Here's how the part is built. I have some questions about the finished solid (model axes, mm). A direction names the side the tool comes from. Round coordinates to 2 decimals unless told otherwise and drop trailing zeros. Order: outer loops, then holes, each group sorted by start corner. A loop starts at its lowest first (then second) coordinate and runs counter-clockwise, first axis right, second up. Notation, with made-up numbers: M -37,63 L 5,63 A14 cw 5,88 Z; hole C 69.25,45 d6. An arc over 180 degrees is marked long. Answer as CSV lines item,"result". Start each with the question number.
```python
from build123d import *

# Parameters (mm, degrees)
SKETCH_1_R          = 5
SKETCH_1_R_2        = 3
EXTRUDE_1_DEPTH     = 12
SKETCH_2_R          = 5.5
CUT_EXTRUDE_1_DEPTH = 6


with BuildPart() as part:
    # 草图1 → 凸台-拉伸1 (new body)
    with BuildSketch(Plane.XY):
        with BuildLine():
            Line((-35, 0), (-35, 35))
            Line((-35, 35), (35, 35))
            Line((35, 35), (35, 0))
            ThreePointArc((35, 0), (0, -35), (-35, 0))
        make_face()
        Circle(SKETCH_1_R, mode=Mode.SUBTRACT)
        with Locations((-27, 29)):
            Circle(SKETCH_1_R_2, mode=Mode.SUBTRACT)
        with Locations((-9, 29)):
            Circle(SKETCH_1_R_2, mode=Mode.SUBTRACT)
        with Locations((9, 29)):
            Circle(SKETCH_1_R_2, mode=Mode.SUBTRACT)
        with Locations((27, 29)):
            Circle(SKETCH_1_R_2, mode=Mode.SUBTRACT)
        with BuildLine():
            ThreePointArc((30, 0), (27, 3), (24, 0))
            ThreePointArc((24, 0), (0, -24), (-24, 0))
            ThreePointArc((-24, 0), (-27, 3), (-30, 0))
            ThreePointArc((-30, 0), (0, -30), (30, 0))
        make_face(mode=Mode.SUBTRACT)
        with BuildLine():
            ThreePointArc((17, 0), (14, 3), (11, 0))
            ThreePointArc((11, 0), (0, -11), (-11, 0))
            ThreePointArc((-11, 0), (-14, 3), (-17, 0))
            ThreePointArc((-17, 0), (0, -17), (17, 0))
        make_face(mode=Mode.SUBTRACT)
    extrude(amount=EXTRUDE_1_DEPTH)

    # 草图2 → 切除-拉伸1 (cut)
    with BuildSketch(Plane.XY.offset(12)):
        with Locations((-27, 29)):
            Circle(SKETCH_2_R)
        with Locations((-9, 29)):
            Circle(SKETCH_2_R)
        with Locations((9, 29)):
            Circle(SKETCH_2_R)
        with Locations((27, 29)):
            Circle(SKETCH_2_R)
        with BuildLine():
            ThreePointArc((32.5, 0), (27, 5.5), (21.5, 0))
            ThreePointArc((21.5, 0), (0, -21.5), (-21.5, 0))
            ThreePointArc((-21.5, 0), (-27, 5.5), (-32.5, 0))
            ThreePointArc((-32.5, 0), (0, -32.5), (32.5, 0))
        make_face()
        with BuildLine():
            ThreePointArc((19.5, 0), (14, 5.5), (8.5, 0))
            ThreePointArc((8.5, 0), (0, -8.5), (-8.5, 0))
            ThreePointArc((-8.5, 0), (-14, 5.5), (-19.5, 0))
            ThreePointArc((-19.5, 0), (0, -19.5), (19.5, 0))
        make_face()
    extrude(amount=-CUT_EXTRUDE_1_DEPTH, mode=Mode.SUBTRACT)


solid = part.part
```
Item 1: If I drill on line 1 along X through (y, z) = (29, 4.5); line 2 along Y through (x, z) = (0, 6.25); line 3 along Y through (x, z) = (0, 3.25), over which ranges is the centre line in solid material (lowest first)?
Item 2: If we section it at C-C on y = -25: Please give me the cut outline in (x, z).
Item 3: If we section it at D-D on y = 29: Count the separate pieces of the cut face and the enclosed holes in it, and give its area (3 significant figures).
Item 4: If we section it at A-A on x = 0: Please give me the cut outline in (y, z).
Item 5: For P1, Ø4, axis at x = -8.5, z = 3, coming from the -Y side; P2, Ø3.5, axis at x = 29, y = 30, coming from the +Z side; P3, Ø6, axis at x = -23, z = 6, coming from the -Y side, each with a flat end and sliding along its axis, tell me the tip position at first contact or that it passes through.
Item 6: We'd pull the mould along X, two halves only. Please class faces 4 (the cylindrical face through (0.528, -23.994, 2.958)), 5 (the flat face through (0, 8, 0)), 6 (the cylindrical face through (0.77, -34.99, 5.92)): pulls with the +X half, pulls with the -X half, needs draft (parallel to the pull), parting line crosses it, or undercut.
Item 7: Which directions (+Z, -Z, +X, -X, +Y, -Y) give clear straight access to the entire face, cutting with the end or side of a thin tool? Please do faces 1 (the cylindrical face through (0, -11, 3)), 2 (the cylindrical face through (-27.716, 34.453, 9.042)), 3 (the flat face through (35, 18, 6)).
Item 8: If we section it at B-B on z = 2.5: Please give me the cut outline in (x, y).
Geometry says:
1,line 1,"-35 to -30, -24 to -12, -6 to 6, 12 to 24, 30 to 35"
1,line 2,"-35 to -32.5, -21.5 to -19.5, -8.5 to -5, 5 to 35"
1,line 3,"-35 to -30, -24 to -17, -11 to -5, 5 to 35"
2,outline,"M -24.49,0 L -16.58,0 L -16.58,6 L -20.77,6 L -20.77,12 L -24.49,12 Z; M 16.58,0 L 24.49,0 L 24.49,12 L 20.77,12 L 20.77,6 L 16.58,6 Z"
3,separate pieces,"5"
3,enclosed holes,"0"
3,area,"432 mm²"
4,outline,"M -35,0 L -30,0 L -30,6 L -32.5,6 L -32.5,12 L -35,12 Z; M -24,0 L -17,0 L -17,6 L -19.5,6 L -19.5,12 L -21.5,12 L -21.5,6 L -24,6 Z; M -11,0 L -5,0 L -5,12 L -8.5,12 L -8.5,6 L -11,6 Z; M 5,0 L 35,0 L 35,12 L 5,12 Z"
5,P1,"y = -34.39"
5,P2,"z = 6"
5,P3,"y = -28.72"
6,face 4,"undercut"
6,face 5,"needs draft"
6,face 6,"parting line crosses it"
7,face 1,"+Z, -Z"
7,face 2,"+Z"
7,face 3,"+Z, -Z, +X, +Y, -Y"
8,outline,"M -35,0 A35 ccw 35,0 L 35,35 L -35,35 Z; hole M -30,0 A30 ccw 30,0 A3 ccw 24,0 A24 cw -24,0 A3 ccw Z; hole C -27,29 d6; hole M -17,0 A17 ccw 17,0 A3 ccw 11,0 A11 cw -11,0 A3 ccw Z; hole C -9,29 d6; hole C 0,0 d10; hole C 9,29 d6; hole C 27,29 d6"
